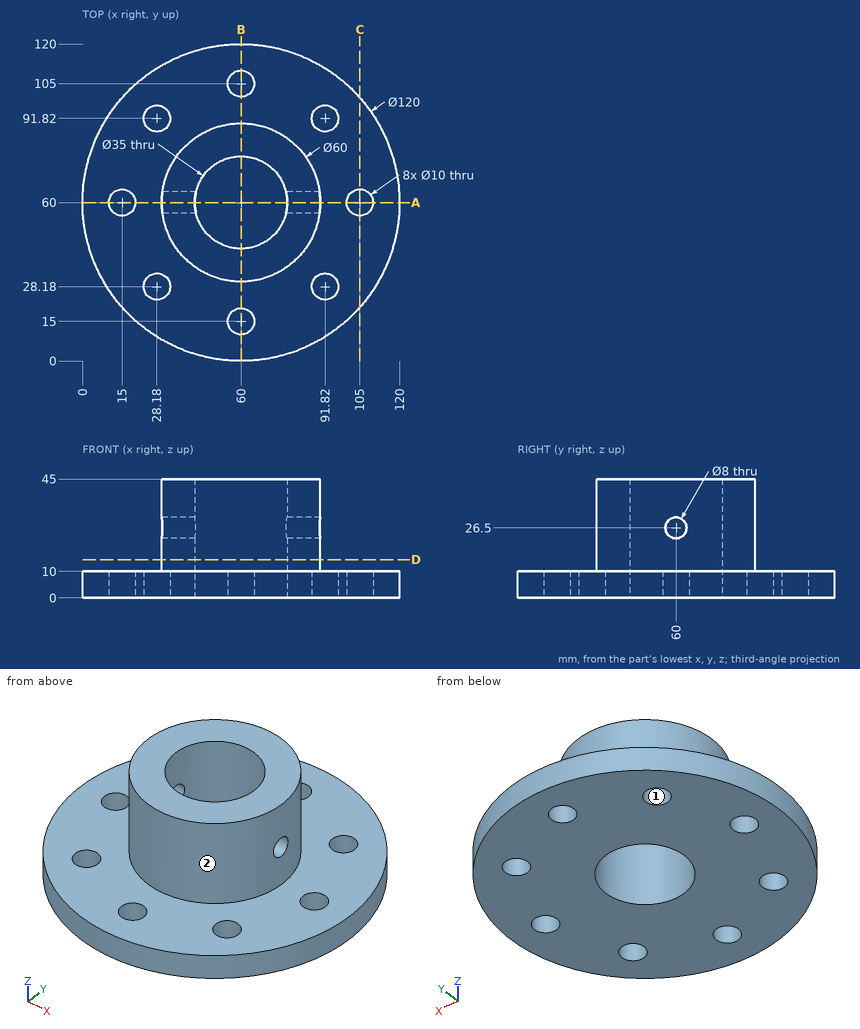
Here's the drawing with two shaded views (mm, measured from the low corner). I have some questions. A direction names the side the tool comes from. Coordinates: 2 decimals unless noted, no trailing zeros. Loops run counter-clockwise (first coordinate to the right, second up) from the corner with the lowest first, then second, coordinate; pieces in that order, holes last. Notation, with made-up numbers: M -38,8.25 L 19,8.25 A9 ccw 19,24.25 Z; hole C 5,-13 d7. An arc over 180 degrees is marked long. Put each result on its own line as item: value. Start each with the question number.
(1) Imagine slicing it at D-D on z = 14.5. List the corners of the cut face in (x, y) for me.
(2) Will these pins go through, and if not, where does the flat tip stop? pin 1 Ø11.5 at (x, y) = (60, 15) entering from +Z; pin 2 Ø10.5 at (y, z) = (60, 26.5) entering from +X; pin 3 Ø10 at (x, z) = (81.5, 32.5) entering from +Y (1 decimal).
(3) Which directions (+Z, -Z, +X, -X, +Y, -Y) give clear straight access to the entire face, cutting with the end or side of a thin tool? Please do the marked faces 1 and 2.
(4) Imagine slicing it at C-C on x = 105. List the corners of the cut face in (y, z) for me, and give its area (3 significant figures).
(5) I need wall thicknesses on probe 1 along Y at (x, z) = (69.5, 22); probe 2 along X at (y, z) = (57, 3.5) (1 decimal); probe 3 along X at (y, z) = (56, 4). Which ranges of each line are inside material? Lowest first, please.
(6) Imagine slicing it at B-B on x = 60. List the corners of the cut face in (y, z) for me.
(7) Imagine slicing it at A-A on y = 60. List the corners of the cut face in (x, z) for me.
Worked answers:
1. outline: C 60,60 d60; hole C 60,60 d35
2. pin 1: stops at z = 10
2. pin 2: stops at x = 90
2. pin 3: stops at y = 85.1
3. face 1: +Z, -Z
3. face 2: +Z
4. outline: M 20.31,0 L 55,0 L 55,10 L 20.31,10 Z; M 65,0 L 99.69,0 L 99.69,10 L 65,10 Z
4. area: 694 mm2
5. probe 1: y = 31.54 to 45.3, 74.7 to 88.46
5. probe 2: x = 0.1 to 11, 19 to 42.8, 77.2 to 101, 109 to 119.9
5. probe 3: x = 0.13 to 12, 18 to 42.96, 77.04 to 102, 108 to 119.87
6. outline: M 0,0 L 10,0 L 10,10 L 0,10 Z; M 20,0 L 42.5,0 L 42.5,45 L 30,45 L 30,10 L 20,10 Z; M 77.5,0 L 100,0 L 100,10 L 90,10 L 90,45 L 77.5,45 Z; M 110,0 L 120,0 L 120,10 L 110,10 Z
7. outline: M 0,0 L 10,0 L 10,10 L 0,10 Z; M 20,0 L 42.5,0 L 42.5,22.5 L 30,22.5 L 30,10 L 20,10 Z; M 30,30.5 L 42.5,30.5 L 42.5,45 L 30,45 Z; M 77.5,0 L 100,0 L 100,10 L 90,10 L 90,22.5 L 77.5,22.5 Z; M 77.5,30.5 L 90,30.5 L 90,45 L 77.5,45 Z; M 110,0 L 120,0 L 120,10 L 110,10 Z
